Source: three-view drawing plus pictorial views. Frame: mm from the lowest corner of the part. A direction names the side the tool comes from. Give positions to 0.01 mm unless a question says otherwise; leave off trailing zeros. Order: outer loops, then holes, each group sorted by start corner. A loop starts at its lowest first (then second) coordinate and runs counter-clockwise, first axis right, second up.
1) Section C-C, the plane x = 23. Give the number of separate pieces and of enclosed holes in the cut face.
2) First-contact query: P1, Ø10, axis at x = 10, y = 30.5, coming from the -Z side; P2, Ø7, axis at x = 14, z = 27, coming from the -Y side; P3, Ø10.5, axis at x = 9.5, y = 12.5, coming from the -Z side; P4, Ø10, axis at x = 10, y = 6.5, coming from the +Z side. Flat tips, straight axial feed; report the tip coordinate or a pass-through.
3) Section D-D, the plane z = 16.5. Return loops of the section in (x, y) (1 decimal), plus the area to 3 significant figures.
4) Draft query along Y for the marked faces 4, 5 and 6. Return one class per face: released by +Y, released by -Y, zero draft, split by the parting line, or undercut.
5) Section B-B, the plane z = 6.5. Return loops of the section in (x, y) (1 decimal).
6) Access query for the marked faces 1, 2 and 3. Directions: +Z, -Z, +X, -X, +Y, -Y. A direction counts if a zero-diameter tool reaches every point of the face in a straight line with its end or side. Return the directions, or none.
7) Material intervals for line 1 (Y direction, x = 1, z = 10.5) (1 decimal); line 2 (Z direction, x = 16.75, y = 7); line 3 (Y direction, x = 23.5, z = 21.75) (1 decimal), sorted ascending.
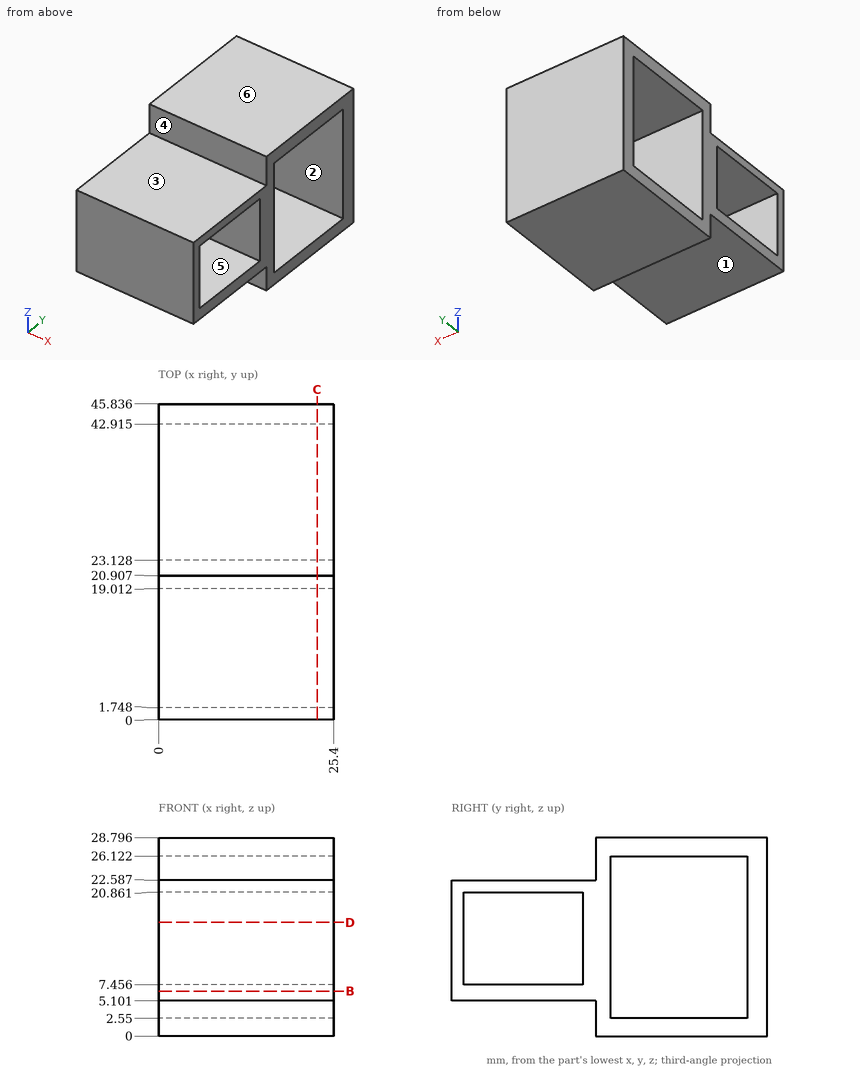
From the geometry:
1. separate pieces: 1
1. enclosed holes: 2
2. P1: stops at z = 0
2. P2: stops at y = 20.91
2. P3: stops at z = 5.1
2. P4: stops at z = 22.59
3. outline: (0, 0) - (25.4, 0) - (25.4, 1.7) - (0, 1.7) - close; (0, 19) - (25.4, 19) - (25.4, 23.1) - (0, 23.1) - close; (0, 42.9) - (25.4, 42.9) - (25.4, 45.8) - (0, 45.8) - close
3. area: 223 mm2
4. face 4: released by -Y
4. face 5: undercut
4. face 6: zero draft
5. outline: (0, 0) - (25.4, 0) - (25.4, 23.1) - (0, 23.1) - close; (0, 42.9) - (25.4, 42.9) - (25.4, 45.8) - (0, 45.8) - close
6. face 1: -Z, +X, -X, -Y
6. face 2: +X, -X
6. face 3: +Z, +X, -X, -Y
7. line 1: y = 0 to 1.7, 19 to 23.1, 42.9 to 45.8
7. line 2: z = 5.1 to 7.46, 20.86 to 22.59
7. line 3: y = 0 to 23.1, 42.9 to 45.8
